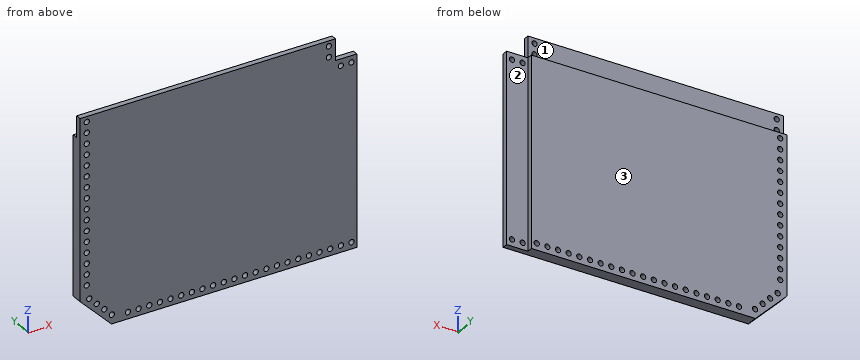
from build123d import *

# Parameters (mm, degrees)
BOSS_EXTRUDE1_DEPTH = 6.35
SKETCH3_R           = 1.5
CUT_EXTRUDE1_DEPTH  = 6.35
LPATTERN2_COUNT     = 22
LPATTERN2_PITCH     = 6.096
SKETCH4_R           = 1.5
CUT_EXTRUDE2_DEPTH  = 6.35
LPATTERN3_COUNT     = 16
LPATTERN3_PITCH     = 6.096
SKETCH6_W           = 120.396
SKETCH6_H           = 3.175
CUT_EXTRUDE3_DEPTH  = 12.192
SKETCH7_W           = 146.304
SKETCH7_H           = 3.175
CUT_EXTRUDE4_DEPTH  = 12.192
SKETCH8_W           = 12.192
SKETCH8_H           = 12.192
CUT_EXTRUDE5_DEPTH  = 6.35
SKETCH9_R           = 1.5
CUT_EXTRUDE6_DEPTH  = 6.35
SKETCH10_R          = 1.5
CUT_EXTRUDE7_DEPTH  = 6.35


with BuildPart() as part:
    # Sketch2 → Boss-Extrude1 (new body)
    with BuildSketch(Plane(origin=(0, 0, 0), x_dir=(1, 0, 0), z_dir=(0, 1, 0))):
        Polygon((-55.206688966, 44.945004491), (-73.167201208, 26.984492248), (-73.167201208, -75.450995509), (85.328798792, -75.450995509), (85.328798792, 44.945004491), align=None)
    extrude(amount=BOSS_EXTRUDE1_DEPTH)

    # Sketch3 → Cut-Extrude1 (cut)
    with BuildSketch(Plane(origin=(0, 6.35, 0), x_dir=(1, 0, 0), z_dir=(0, 1, 0))):
        with Locations(Location((82.280798792, 41.135004491, 0), (0, 0, 270))):
            Circle(SKETCH3_R)
    cut_extrude1 = extrude(amount=-CUT_EXTRUDE1_DEPTH, mode=Mode.SUBTRACT)

    # LPattern2: Cut-Extrude1 ×22
    with Locations(*[(-i * LPATTERN2_PITCH, 0, 0) for i in range(1, LPATTERN2_COUNT)]):
        add(cut_extrude1, mode=Mode.SUBTRACT)

    # Sketch4 → Cut-Extrude2 (cut)
    with BuildSketch(Plane(origin=(0, 6.35, 0), x_dir=(1, 0, 0), z_dir=(0, 1, 0))):
        with Locations(Location((-69.357201208, -72.402995509, 0), (0, 0, 270))):
            Circle(SKETCH4_R)
    cut_extrude2 = extrude(amount=-CUT_EXTRUDE2_DEPTH, mode=Mode.SUBTRACT)

    # LPattern3: Cut-Extrude2 ×16
    with Locations(*[(0, 0, -i * LPATTERN3_PITCH) for i in range(1, LPATTERN3_COUNT)]):
        add(cut_extrude2, mode=Mode.SUBTRACT)

    # Sketch6 → Cut-Extrude3 (cut)
    with BuildSketch(Plane(origin=(85.328798792, 0, 0), x_dir=(0, 0, -1), z_dir=(1, 0, 0))):
        with Locations((-15.252995509, 4.7625)):
            Rectangle(SKETCH6_W, SKETCH6_H)
    extrude(amount=-CUT_EXTRUDE3_DEPTH, mode=Mode.SUBTRACT)

    # Sketch7 → Cut-Extrude4 (cut)
    with BuildSketch(Plane.XY.offset(75.450995509)):
        with Locations((-0.015201208, 4.7625)):
            Rectangle(SKETCH7_W, SKETCH7_H)
    extrude(amount=-CUT_EXTRUDE4_DEPTH, mode=Mode.SUBTRACT)

    # Sketch8 → Cut-Extrude5 (cut)
    with BuildSketch(Plane(origin=(0, 3.175, 0), x_dir=(1, 0, 0), z_dir=(0, 1, 0))):
        with Locations((79.232798792, -69.354995509)):
            Rectangle(SKETCH8_W, SKETCH8_H)
    extrude(amount=-CUT_EXTRUDE5_DEPTH, mode=Mode.SUBTRACT)

    # Sketch9 → Cut-Extrude6 (cut)
    with BuildSketch(Plane(origin=(0, 3.175, 0), x_dir=(1, 0, 0), z_dir=(0, 1, 0))):
        with Locations(Location((69.326798792, -66.306995509, 0), (0, 0, 270))):
            Circle(SKETCH9_R)
        with Locations(Location((69.326798792, -72.402995509, 0), (0, 0, 270))):
            Circle(SKETCH9_R)
        with Locations(Location((76.184798792, -59.448995509, 0), (0, 0, 270))):
            Circle(SKETCH9_R)
        with Locations(Location((82.280798792, -59.448995509, 0), (0, 0, 270))):
            Circle(SKETCH9_R)
    extrude(amount=-CUT_EXTRUDE6_DEPTH, mode=Mode.SUBTRACT)

    # Sketch10 → Cut-Extrude7 (cut)
    with BuildSketch(Plane(origin=(0, 6.35, 0), x_dir=(1, 0, 0), z_dir=(0, 1, 0))):
        with Locations(Location((-59.294699493, 35.46884029, 0), (0, 0, 270))):
            Circle(SKETCH10_R)
        with Locations(Location((-63.605762233, 31.157777551, 0), (0, 0, 270))):
            Circle(SKETCH10_R)
        with Locations(Location((-54.984176555, 39.779363228, 0), (0, 0, 270))):
            Circle(SKETCH10_R)
        with Locations(Location((-67.916285171, 26.847254613, 0), (0, 0, 270))):
            Circle(SKETCH10_R)
    extrude(amount=-CUT_EXTRUDE7_DEPTH, mode=Mode.SUBTRACT)


solid = part.part
Could you check a few things on this model? Use its own coordinates, in mm. Face numbers are marked on the shaded views. A direction names the side the tool comes from. Coordinates: 2 decimals unless noted, no trailing zeros. One line per item, written item: value. Start each with the question number.
1) Imagine slicing it at A-A on y = 4.5. Count the separate pieces of the cut face and the enclosed holes in it, plus the area to 3 significant figures.
2) I'm going to push a flat-ended pin straight in: pin 1 (3.5 mm diameter, centred on x = 69.33, z = 66.31, fed in from +Y) (3 decimals). Where does the tip first touch, or does it pass through?
3) Which directions (+Z, -Z, +X, -X, +Y, -Y) give clear straight access to the entire face, cutting with the end or side of a thin tool? Please do the marked faces 1, 2 and 3.
4) If I drill on L1, parallel to X at y = 1, z = -6.5; L2, parallel to Z at x = -15, y = 3 (3 decimals); L3, parallel to Z at x = -9.5, y = 6 (3 decimals), over which ranges is the centre line in solid material (lowest first)? Write a range as [from, to].
Answer list:
1. separate pieces: 1
1. enclosed holes: 38
1. area: 15,400 mm2
2. pin 1: stops at y = 3.175
3. face 1: +Z, +X, -X, +Y
3. face 2: +Z, -Z, +X, +Y
3. face 3: +Z, -Z, +X, -X, +Y
4. L1: x = [-73.17, -70.82], [-67.9, 85.33]
4. L2: z = [-44.945, -42.613], [-39.657, 75.451]
4. L3: z = [-44.945, -42.596], [-39.674, 63.259]
